```python
from build123d import *

# Parameters (mm, degrees)
EXTRUDE_1_DEPTH     = 100
SKETCH_2_R          = 2.5
CUT_EXTRUDE_1_DEPTH = 100
SKETCH_3_R          = 3.25
SKETCH_3_R_2        = 1.75
EXTRUDE_2_DEPTH     = 5
SKETCH_4_R          = 1.75
CUT_EXTRUDE_3_DEPTH = 5
SKETCH_5_R          = 3.25
SKETCH_5_R_2        = 1.75
EXTRUDE_3_DEPTH     = 5
SKETCH_6_R          = 1.75
CUT_EXTRUDE_4_DEPTH = 5


with BuildPart() as part:
    # 草图1 → 凸台-拉伸1 (new body)
    with BuildSketch(Plane.XY):
        Polygon((0, 7.1), (50, 57.1), (100, 7.1), (92.928932188, 7.1), (50, 50.028932188), (7.071067812, 7.1), align=None)
    extrude(amount=EXTRUDE_1_DEPTH)

    # 草图2 → 切除-拉伸1 (cut)
    with BuildSketch(Plane(origin=(53.55, 53.55, 0), x_dir=(0, 0, -1), z_dir=(0.7071067811865474, 0.7071067811865477, 0))):
        with Locations(Location((-50, -15.334880913, 0), (0, 0, 90))):
            Circle(SKETCH_2_R)
        with Locations(Location((-50, -45.334880913, 0), (0, 0, 90))):
            Circle(SKETCH_2_R)
    extrude(amount=-CUT_EXTRUDE_1_DEPTH, mode=Mode.SUBTRACT)

    # 草图3 → 凸台-拉伸2 (add)
    # profile 1 of 2: a face of its own
    with BuildSketch(Plane.XZ.offset(-7.1)):
        with Locations((96.464466094, 90)):
            Circle(SKETCH_3_R)
        with Locations((96.464466094, 90)):
            Circle(SKETCH_3_R_2, mode=Mode.SUBTRACT)
    # profile 2 of 2: a face of its own
    with BuildSketch(Plane.XZ.offset(-7.1)):
        with Locations((96.464466094, 10)):
            Circle(SKETCH_3_R)
        with Locations((96.464466094, 10)):
            Circle(SKETCH_3_R_2, mode=Mode.SUBTRACT)
    extrude(amount=-EXTRUDE_2_DEPTH)

    # 草图4 → 切除-拉伸3 (cut)
    with BuildSketch(Plane.XZ.offset(-7.1)):
        with Locations((96.464466094, 90)):
            Circle(SKETCH_4_R)
        with Locations((96.464466094, 10)):
            Circle(SKETCH_4_R)
    extrude(amount=-CUT_EXTRUDE_3_DEPTH, mode=Mode.SUBTRACT)

    # 草图5 → 凸台-拉伸3 (add)
    # profile 1 of 2: a face of its own
    with BuildSketch(Plane.XZ.offset(-7.1)):
        with Locations((3.535533906, 90)):
            Circle(SKETCH_5_R)
        with Locations((3.535533906, 90)):
            Circle(SKETCH_5_R_2, mode=Mode.SUBTRACT)
    # profile 2 of 2: a face of its own
    with BuildSketch(Plane.XZ.offset(-7.1)):
        with Locations((3.535533906, 10)):
            Circle(SKETCH_5_R)
        with Locations((3.535533906, 10)):
            Circle(SKETCH_5_R_2, mode=Mode.SUBTRACT)
    extrude(amount=-EXTRUDE_3_DEPTH)

    # 草图6 → 切除-拉伸4 (cut)
    with BuildSketch(Plane.XZ.offset(-7.1)):
        with Locations((3.535533906, 10)):
            Circle(SKETCH_6_R)
        with Locations((3.535533906, 90)):
            Circle(SKETCH_6_R)
    extrude(amount=-CUT_EXTRUDE_4_DEPTH, mode=Mode.SUBTRACT)


solid = part.part
```
CAD build for the part. Positions are in the model's coordinates, mm. A direction names the side the tool comes from. Coordinates: 2 decimals unless noted, no trailing zeros. Order: outer loops, then holes, each group sorted by start corner. A loop starts at its lowest first (then second) coordinate and runs counter-clockwise, first axis right, second up.
(1) Saw through at B-B, the plane z = 18. Write the cut outline in (x, y).
Solution:
outline: (0, 7.1) - (7.07, 7.1) - (50, 50.03) - (92.93, 7.1) - (100, 7.1) - (50, 57.1) - close
(2) Saw through at A-A, the plane y = 47. Write the cut outline in (x, z).
Solution:
outline: (39.9, 0) - (46.97, 0) - (46.97, 100) - (39.9, 100) - close; (53.03, 0) - (60.1, 0) - (60.1, 100) - (53.03, 100) - close
(3) Drill centre lines: L1, parallel to Z at x = 84, y = 17.5; L2, parallel to X at y = 37.5, z = 16; L3, parallel to X at y = 48.5, z = 76.5. Where is each one in solid material? Low to high.
Solution:
L1: z = 0 to 48.16, 51.84 to 100
L2: x = 30.4 to 37.47, 62.53 to 69.6
L3: x = 41.4 to 48.47, 51.53 to 58.6
(4) Pin check, flat tips, straight feed: pin 1 Ø5 at (x, z) = (3, 90) entering from +Y; pin 2 Ø8 at (y, z) = (49, 27.5) entering from +X; pin 3 Ø2.5 at (x, z) = (97, 91) entering from +Y. Stop position of each tip, or through.
Solution:
pin 1: stops at y = 12.6
pin 2: stops at x = 62.1
pin 3: stops at y = 12.1
(5) Which spindle directions (+Z, -Z, +X, -X, +Y, -Y) get a long thin tool onto all of the face, cutting with end or side? Do faces 1 (the face through (98.4, 12.1, 90)), 2 (the face through (96, 7.1, 51)), 3 (the face through (71.765, 28.264, 49.3)), 4 (the face through (61, 40, 100)), 5 (the face through (1.6, 12.1, 90)). Say none if no direction does.
Solution:
face 1: +Z, -Z, +X, +Y
face 2: +Z, -Z, +X, -X, -Y
face 3: +Z, -Z, -Y
face 4: +Z, +X, -X, +Y, -Y
face 5: +Z, -Z, -X, +Y
(6) Mould opens along Y. For faces 6 (the face through (28.836, 28.865, 49.3)), 7 (the face through (61, 40, 0)), 8 (the face through (82.18, 21.44, 50.75)), 9 (the face through (1.6, 12.1, 10)) say: released by +Y, released by -Y, zero draft, split by the parting line, or undercut.
Solution:
face 6: released by -Y
face 7: zero draft
face 8: undercut
face 9: released by +Y
(7) Saw through at C-C, the plane x = 46.5. Write the cut outline in (y, z), and give its area (3 significant figures).
Solution:
outline: (46.53, 0) - (53.6, 0) - (53.6, 100) - (46.53, 100) - close
area: 707 mm2
